Could you check a few things on this drawing? It's one solid part, dimensions in mm from its lowest x, y, z. A direction names the side the tool comes from. Give positions to 0.01 mm unless a question says otherwise; leave off trailing zeros. Loops run counter-clockwise (first coordinate to the right, second up) from the corner with the lowest first, then second, coordinate; pieces in that order, holes last. Notation, with made-up numbers: M 36.25,-7 L 44.25,-7 A21 ccw 44.25,29 Z; hole C -11.75,2 d5. An arc over 180 degrees is marked long. Answer in a Markdown table with one row per item. Add a question column.
1. I need wall thicknesses on line 1 along Y through (x, z) = (6, 3.8); line 2 along Y through (x, z) = (6, 1.1); line 3 along Z through (x, y) = (2.5, 6.5). Which ranges of each line are inside material? Lowest first, please. Write a range as from..to.
2. If we section it at A-A on y = 6: List the corners of the cut face in (x, z) for me.
3. If we section it at D-D on y = 9: List the corners of the cut face in (x, z) for me.
4. If we section it at C-C on z = 0.4: List the corners of the cut face in (x, y) for me.
5. Thinking about a two-plate mould opening in Y: for the marked faces 1, 2 and 3, which applies, released by +Y, released by -Y, zero draft, split by the parting line, or undercut?
6. I'm going to push flat-ended pins straight in: pin 1 Ø4 at (x, y) = (6.5, 3.5) entering from +Z; pin 2 Ø3 at (x, y) = (6, 6) entering from -Z; pin 3 Ø3 at (y, z) = (9, 1.5) entering from +X; pin 4 Ø6.5 at (x, y) = (6, 6) entering from +Z. Where does each tip first touch, or does it pass through?
7. Which directions (+Z, -Z, +X, -X, +Y, -Y) give clear straight access to the entire face, cutting with the end or side of a thin tool? Please do the marked faces 4 and 5.
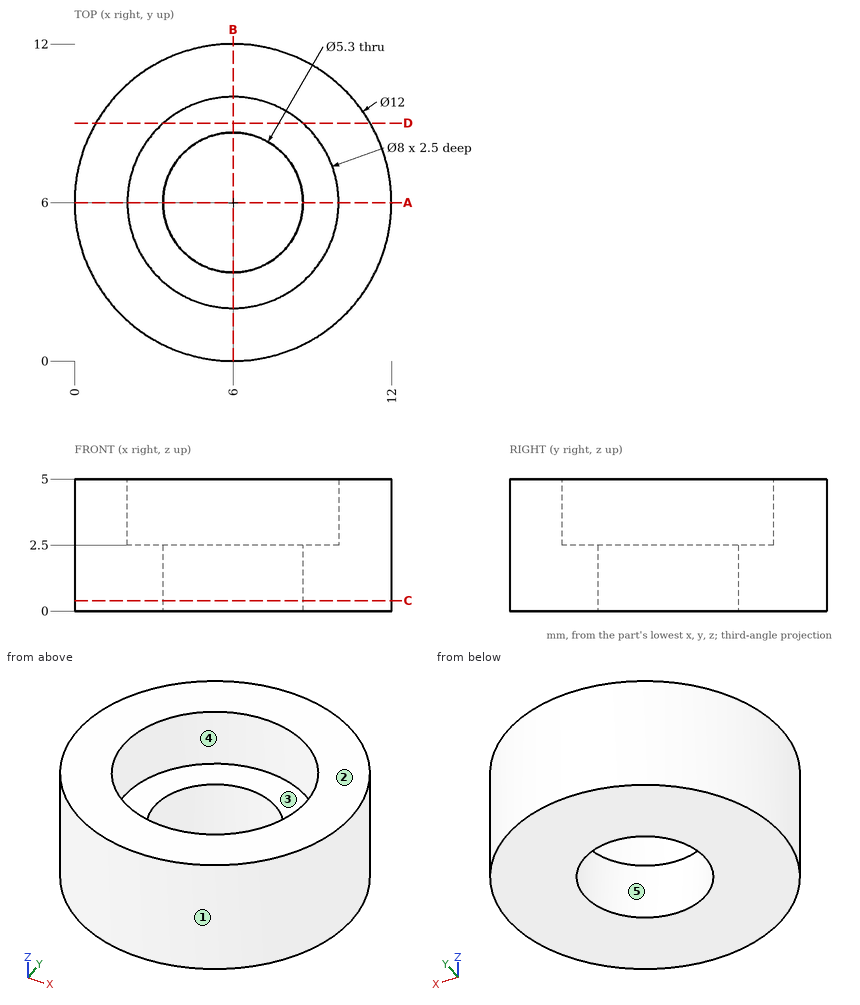
Results:
| question | item | result |
|---|---|---|
| 1 | line 1 | 0..2, 10..12 |
| 1 | line 2 | 0..3.35, 8.65..12 |
| 1 | line 3 | 0..2.5 |
| 2 | outline | M 0,0 L 3.35,0 L 3.35,2.5 L 2,2.5 L 2,5 L 0,5 Z; M 8.65,0 L 12,0 L 12,5 L 10,5 L 10,2.5 L 8.65,2.5 Z |
| 3 | outline | M 0.8,0 L 11.2,0 L 11.2,5 L 8.65,5 L 8.65,2.5 L 3.35,2.5 L 3.35,5 L 0.8,5 Z |
| 4 | outline | C 6,6 d12; hole C 6,6 d5.3 |
| 5 | face 1 | split by the parting line |
| 5 | face 2 | zero draft |
| 5 | face 3 | undercut |
| 6 | pin 1 | z = 5 |
| 6 | pin 2 | through |
| 6 | pin 3 | x = 11.81 |
| 6 | pin 4 | z = 2.5 |
| 7 | face 4 | +Z |
| 7 | face 5 | +Z, -Z |
